```python
from build123d import *

# Parameters (mm, degrees)
F0_W      = 762
F0_H      = 457.2
F1_DEPTH  = 50.8
F0_W_2    = 1422.4
F0_H_2    = 1016
F1_FACE_W = 762
F1_FACE_H = 457.2
F2_DEPTH  = 25.4
F3_R      = 12.7


with BuildPart() as f1:
    # F0 (on Front) → F1 (new body)
    with BuildSketch(Plane.XZ):
        with Locations((0, -177.8)):
            Rectangle(F0_W, F0_H)
    extrude(amount=-F1_DEPTH)

    # F0 (on Front) + F1_face (on face) → F2 (join)
    with BuildSketch(Plane.XZ):
        Rectangle(F0_W_2, F0_H_2)
        with Locations((0, -177.8)):
            Rectangle(F0_W, F0_H, mode=Mode.SUBTRACT)
    with BuildSketch(Plane(origin=(0, 0, -177.8), x_dir=(1, 0, 0), z_dir=(0, -1, 0))):
        Rectangle(F1_FACE_W, F1_FACE_H)
    extrude(amount=F2_DEPTH)

    # F3
    f3_edges = [f1.edges().sort_by_distance(p)[0] for p in [
        (711.2, -12.7, -508),
        (-711.2, -12.7, -508),
        (-711.2, -12.7, 508),
        (711.2, -12.7, 508),
    ]]
    fillet(f3_edges, radius=F3_R)


solid = f1.part
```
Geometry: final body of the model. Coordinates: model frame, mm. A direction names the side the tool comes from. Round coordinates to 2 decimals unless told otherwise and drop trailing zeros. Write each loop counter-clockwise with the first axis right and the second up, starting at its lowest first coordinate (ties: lowest second). Pieces come first, ordered by that corner, then holes.
Item 1: Section query B-B (x = 267). Return loops of the section in (y, z).
Item 2: Material intervals for L1, parallel to Y at x = -57, z = 336; L2, parallel to Z at x = -370, y = 17.5; L3, parallel to X at y = 8, z = 25, sorted ascending.
Item 3: Set-up query: faces 1 (the face through (-5, 25, 50.8)), 2 (the face through (-381, 25, -181)), 3 (the face through (-5, 25, -406.4)), 4 (the face through (381, 25, -181)). Return all of +Z, -Z, +X, -X, +Y, -Y with unobstructed straight access to the full face (end or side cutting, diameter ignored); none if empty.
Item 4: Section query D-D (z = 281). Return loops of the section in (x, y).
Item 5: Pin query (flat end, axial travel): P1, Ø1.5, axis at x = 32, z = 278.5, coming from the +Y side; P2, Ø1.5, axis at y = 37.5, z = 31, coming from the -X side; P3, Ø15, axis at x = -111, y = 25.5, coming from the +Z side. Return the tip coordinate at first contact, or that it passes through.
Item 6: Section query C-C (y = 28). Return loops of the section in (x, z).
Item 7: Section query A-A (z = -291.5). Return loops of the section in (x, y).
Completed:
1. outline: (-25.4, -508) - (0, -508) - (0, -406.4) - (50.8, -406.4) - (50.8, 50.8) - (0, 50.8) - (0, 508) - (-25.4, 508) - close
2. L1: y = -25.4 to 0
2. L2: z = -406.4 to 50.8
2. L3: x = -381 to 381
3. face 1: +Z, +X, -X, +Y
3. face 2: +Z, -Z, -X, +Y
3. face 3: -Z, +X, -X, +Y
3. face 4: +Z, -Z, +X, +Y
4. outline: (-711.2, -25.4) - (711.2, -25.4) - (711.2, 0) - (-711.2, 0) - close
5. P1: stops at y = 0
5. P2: stops at x = -381
5. P3: stops at z = 50.8
6. outline: (-381, -406.4) - (381, -406.4) - (381, 50.8) - (-381, 50.8) - close
7. outline: (-711.2, -25.4) - (711.2, -25.4) - (711.2, 0) - (381, 0) - (381, 50.8) - (-381, 50.8) - (-381, 0) - (-711.2, 0) - close
